Source: CAD feature listing. Evaluate the final solid. Frame: model axes, mm. A direction names the side the tool comes from. Round coordinates to 2 decimals unless told otherwise and drop trailing zeros. Write each loop counter-clockwise with the first axis right and the second up, starting at its lowest first coordinate (ties: lowest second). Pieces come first, ordered by that corner, then holes. Notation, with made-up numbers: (31.25, -2.75) - (76.25, -2.75) arc R9 cw to (76.25, 13.25) - close; hole circle Ø4 at (24.25, 60.25). An arc over 180 degrees is marked (long way). Write item = value, one per line. Start each with the question number.
```python
from build123d import *

# Parameters (mm, degrees)
SKETCH_1_R          = 2.5
EXTRUDE_1_DEPTH     = 200
CUT_EXTRUDE_6_DEPTH = 90
CUT_EXTRUDE_7_DEPTH = 203.263183999


with BuildPart() as part:
    # 草图1 → 凸台-拉伸1 (new body)
    with BuildSketch(Plane(origin=(0, 0, 0), x_dir=(1, 0, 0), z_dir=(0, 1, 0))):
        with BuildLine():
            Line((-20.885583918, -15.691936644), (-22.685583918, -15.691936644))
            Line((-22.685583918, -15.691936644), (-22.685583918, -21.091936644))
            ThreePointArc((-22.685583918, -21.091936644), (-22.24624409, -22.152596816), (-21.185583918, -22.591936644))
            Line((-21.185583918, -22.591936644), (-15.785583918, -22.591936644))
            Line((-15.785583918, -22.591936644), (-15.785583918, -20.791936644))
            Line((-15.785583918, -20.791936644), (-18.185583918, -20.791936644))
            Line((-18.185583918, -20.791936644), (-18.185583918, -18.988986799))
            Line((-18.185583918, -18.988986799), (-14.888533763, -15.691936644))
            Line((-14.888533763, -15.691936644), (-10.482634073, -15.691936644))
            Line((-10.482634073, -15.691936644), (-7.185583918, -18.988986799))
            Line((-7.185583918, -18.988986799), (-7.185583918, -20.791936644))
            Line((-7.185583918, -20.791936644), (-9.585583918, -20.791936644))
            Line((-9.585583918, -20.791936644), (-9.585583918, -22.591936644))
            Line((-9.585583918, -22.591936644), (-4.185583918, -22.591936644))
            ThreePointArc((-4.185583918, -22.591936644), (-3.124923747, -22.152596816), (-2.685583918, -21.091936644))
            Line((-2.685583918, -21.091936644), (-2.685583918, -15.691936644))
            Line((-2.685583918, -15.691936644), (-4.485583918, -15.691936644))
            Line((-4.485583918, -15.691936644), (-4.485583918, -18.091936644))
            Line((-4.485583918, -18.091936644), (-6.288533763, -18.091936644))
            Line((-6.288533763, -18.091936644), (-9.631456898, -14.749013509))
            Line((-9.631456898, -14.749013509), (-9.631456898, -10.434859779))
            Line((-9.631456898, -10.434859779), (-6.288533763, -7.091936644))
            Line((-6.288533763, -7.091936644), (-4.485583918, -7.091936644))
            Line((-4.485583918, -7.091936644), (-4.485583918, -9.491936644))
            Line((-4.485583918, -9.491936644), (-2.685583918, -9.491936644))
            Line((-2.685583918, -9.491936644), (-2.685583918, -4.091936644))
            ThreePointArc((-2.685583918, -4.091936644), (-3.124923747, -3.031276473), (-4.185583918, -2.591936644))
            Line((-4.185583918, -2.591936644), (-9.585583918, -2.591936644))
            Line((-9.585583918, -2.591936644), (-9.585583918, -4.391936644))
            Line((-9.585583918, -4.391936644), (-7.185583918, -4.391936644))
            Line((-7.185583918, -4.391936644), (-7.185583918, -6.194886489))
            Line((-7.185583918, -6.194886489), (-10.482634073, -9.491936644))
            Line((-10.482634073, -9.491936644), (-14.888533763, -9.491936644))
            Line((-14.888533763, -9.491936644), (-18.185583918, -6.194886489))
            Line((-18.185583918, -6.194886489), (-18.185583918, -4.391936644))
            Line((-18.185583918, -4.391936644), (-15.785583918, -4.391936644))
            Line((-15.785583918, -4.391936644), (-15.785583918, -2.591936644))
            Line((-15.785583918, -2.591936644), (-21.185583918, -2.591936644))
            ThreePointArc((-21.185583918, -2.591936644), (-22.24624409, -3.031276473), (-22.685583918, -4.091936644))
            Line((-22.685583918, -4.091936644), (-22.685583918, -9.491936644))
            Line((-22.685583918, -9.491936644), (-20.885583918, -9.491936644))
            Line((-20.885583918, -9.491936644), (-20.885583918, -7.091936644))
            Line((-20.885583918, -7.091936644), (-19.082634073, -7.091936644))
            Line((-19.082634073, -7.091936644), (-15.739710939, -10.434859779))
            Line((-15.739710939, -10.434859779), (-15.739710939, -14.749013509))
            Line((-15.739710939, -14.749013509), (-19.082634073, -18.091936644))
            Line((-19.082634073, -18.091936644), (-20.885583918, -18.091936644))
            Line((-20.885583918, -18.091936644), (-20.885583918, -15.691936644))
        make_face()
        with Locations(Location((-12.685583918, -12.591936644, 0), (0, 0, 270))):
            Circle(SKETCH_1_R, mode=Mode.SUBTRACT)
    extrude(amount=EXTRUDE_1_DEPTH)

    # 草图4 → 切除-拉伸6 (cut)
    with BuildSketch(Plane.ZY.offset(22.685583918)):
        Polygon((22.591936644, 200), (2.591936644, 180), (2.591936644, 200), align=None)
    extrude(amount=-CUT_EXTRUDE_6_DEPTH, mode=Mode.SUBTRACT)

    # 草图5 → 切除-拉伸7 (cut, through all)
    with BuildSketch(Plane.ZY.offset(22.685583918)):
        Polygon((2.591936644, 0), (22.591936644, 20), (22.591936644, 0), align=None)
    extrude(amount=-CUT_EXTRUDE_7_DEPTH, mode=Mode.SUBTRACT)


solid = part.part
```
(1) Section A-A (z = 13). Return the cut outline in (x, y), plus the area to 3 significant figures.
(2) Ray query, L1, parallel to X at y = 117, z = 20; L2, parallel to Z at x = -20, y = 149; L3, parallel to X at y = 62, z = 8.25. Return the intervals inside material, ascending. Write a range as from..to.
(3) Pull-direction query (Z, two-part tool) for faces 5 (the flat face through (-10.6, 12.08, 14.67)), 6 (the flat face through (-16.51, 93.97, 7.87)), 7 (the flat face through (-18, 89, 2.592)); classes: +Z half, -Z half, draft (parallel to the pull), parting line (faces both ways), or undercut.
(4) Contact query for flat-ended pins moving along their axis: P1, Ø2, axis at y = 120, z = 21.5, coming from the -X side; P2, Ø1.4, axis at y = 58.5, z = 3, coming from the -X side; P3, Ø4, axis at x = -7, z = 5, coming from the -Y side; P4, Ø6, axis at x = -14.5, z = 14.5, coming from the -Y side. Output: stop coordinate, or through.
(5) Reachability of faces 1 (the flat face through (-13, 102, 15.692)), 2 (the flat face through (-9.631, 99, 13)), 3 (the flat face through (-8.857, 103.465, 17.317)), 4 (the flat face through (-13, 96, 9.492)) from +Z, -Z, +X, -X, +Y, -Y: full face, straight path, thin tool, end or side. Return the list, or none.
Solution:
q1.outline = (-15.74, 10.41) - (-15.15, 10.41) - (-15.15, 190.41) - (-15.74, 190.41) - close; (-10.22, 10.41) - (-9.63, 10.41) - (-9.63, 190.41) - (-10.22, 190.41) - close
q1.area = 212 mm^2
q2.L1 = -22.69..-18.19, -7.19..-2.69
q2.L2 = 2.59..7.09, 18.09..22.59
q2.L3 = -22.69..-20.89, -17.92..-16.13, -9.24..-7.45, -4.49..-2.69
q3.face_5 = +Z half
q3.face_6 = undercut
q3.face_7 = -Z half
q4.P1 = -22.69
q4.P2 = -22.63
q4.P3 = 0.41
q4.P4 = 8.94
q5.face_1 = +Z, +Y, -Y
q5.face_2 = +X, +Y, -Y
q5.face_3 = +Y, -Y
q5.face_4 = -Z, +Y, -Y
